```python
from build123d import *

# Parameters (mm, degrees)
SKETCH_1_R      = 3.4455
EXTRUDE_1_DEPTH = 6.8
CHAMFER_1_SIZE  = 0.5545


with BuildPart() as part:
    # Эскиз1 → Бобышка-Вытянуть1 (new body)
    with BuildSketch(Plane.XY):
        Polygon((0, 7.505553499), (-6.5, 3.75277675), (-6.5, -3.75277675), (0, -7.505553499), (6.5, -3.75277675), (6.5, 3.75277675), align=None)
        Circle(SKETCH_1_R, mode=Mode.SUBTRACT)
    extrude(amount=EXTRUDE_1_DEPTH)

    # Фаска1
    chamfer_1_edges = [part.edges().sort_by_distance(p)[0] for p in [
        (-3.4455, 0, 0),
        (-3.4455, 0, 6.8),
    ]]
    chamfer(chamfer_1_edges, length=CHAMFER_1_SIZE)


solid = part.part
```
Could you check a few things on this model? Use its own coordinates, in mm. Round coordinates to 2 decimals unless told otherwise and drop trailing zeros. Loops run counter-clockwise (first coordinate to the right, second up) from the corner with the lowest first, then second, coordinate; pieces in that order, holes last.
Q1. For P1, Ø4, axis at x = 2.5, z = 3, coming from the +Y side; P2, Ø6, axis at x = 0, y = 0, coming from the +Z side, each with a flat end and sliding along its axis, tell me the tip position at first contact or that it passes through.
Q2. Please list where these lines run through material, in increasing order: L1, parallel to X at y = 1.25, z = 3; L2, parallel to Y at x = -2.75, z = 6; L3, parallel to Y at x = 4.75, z = 2.
Q3. I want a section at D-D (x = -5.5). Write out the boundary of the cut face in (y, z), and give its area (3 significant figures).
Q4. I want a section at A-A (y = 0). Write out the boundary of the cut face in (x, z).
Q5. I want a section at B-B (z = 0.75). Write out the boundary of the cut face in (x, y), and give its area (3 significant figures).
Q6. I want a section at C-C (y = -4.5). Write out the boundary of the cut face in (x, z), and give its area (3 significant figures).
Q7. Thinking about a two-plate mould opening in Y: for faces 1 (the flat face through (-6.5, 0, 3)), 2 (the flat face through (3.2, -5.66, 3.35)), 3 (the flat face through (-3.2, 5.66, 3.35)), 4 (the cylindrical face through (-0.747, -3.364, 3.36)), which applies, pulls with the +Y half, pulls with the -Y half, needs draft (parallel to the pull), parting line crosses it, or undercut?
Answer below:
1. P1: stops at y = 7.22
1. P2: passes through
2. L1: x = -6.5 to -3.21, 3.21 to 6.5
2. L2: y = -5.92 to -2.08, 2.08 to 5.92
2. L3: y = -4.76 to 4.76
3. outline: (-4.33, 0) - (4.33, 0) - (4.33, 6.8) - (-4.33, 6.8) - close
3. area: 58.9 mm2
4. outline: (-6.5, 0) - (-4, 0) - (-3.45, 0.55) - (-3.45, 6.25) - (-4, 6.8) - (-6.5, 6.8) - close; (3.45, 0.55) - (4, 0) - (6.5, 0) - (6.5, 6.8) - (4, 6.8) - (3.45, 6.25) - close
5. outline: (-6.5, -3.75) - (0, -7.51) - (6.5, -3.75) - (6.5, 3.75) - (0, 7.51) - (-6.5, 3.75) - close; hole circle Ø6.89 at (0, 0)
5. area: 109 mm2
6. outline: (-5.21, 0) - (5.21, 0) - (5.21, 6.8) - (-5.21, 6.8) - close
6. area: 70.8 mm2
7. face 1: needs draft
7. face 2: pulls with the -Y half
7. face 3: pulls with the +Y half
7. face 4: undercut
